```python
from build123d import *

# Parameters (mm, degrees)
F0_W     = 45.3136
F0_H     = 45.3136
F1_DEPTH = 2.3876
F2_R     = 22.6568
F2_R_2   = 19.8374
F3_DEPTH = 92.2274
F4_W     = 28.575
F4_H     = 28.575
F5_DEPTH = 4.7752
F6_R     = 21.1328
F7_DEPTH = 19.05
F8_R     = 5.08


with BuildPart() as f1:
    # F0 (on Top) → F1 (new body, symmetric)
    with BuildSketch(Plane.XY):
        Rectangle(F0_W, F0_H)
    extrude(amount=F1_DEPTH, both=True)

    # F2 (on face) → F3 (join)
    with BuildSketch(Plane.XY.offset(2.3876)):
        Circle(F2_R)
        Circle(F2_R_2, mode=Mode.SUBTRACT)
    extrude(amount=F3_DEPTH)

    # F4 (on face) → F5 (cut, through all)
    with BuildSketch(Plane(origin=(0, 0, -2.3876), x_dir=(1, 0, 0), z_dir=(0, 0, -1))):
        Rectangle(F4_W, F4_H)
    extrude(amount=-F5_DEPTH, mode=Mode.SUBTRACT)

    # F6 (on face) → F7 (cut)
    with BuildSketch(Plane.XY.offset(94.615)):
        Circle(F6_R)
    extrude(amount=-F7_DEPTH, mode=Mode.SUBTRACT)

    # F8
    f8_edges = [f1.edges().sort_by_distance(p)[0] for p in [
        (-22.6568, -22.6568, 0),
        (-22.6568, 22.6568, 0),
        (22.6568, -22.6568, 0),
        (22.6568, 22.6568, 0),
    ]]
    fillet(f8_edges, radius=F8_R)


solid = f1.part
```
Check sheet for the modelled part. Datum: model origin and axes. Units: mm. A direction names the side the tool comes from. Round coordinates to 2 decimals unless told otherwise and drop trailing zeros. Write each loop counter-clockwise with the first axis right and the second up, starting at its lowest first coordinate (ties: lowest second). Pieces come first, ordered by that corner, then holes. Notation, with made-up numbers: (28, 79.25) -> (36, 79.25) arc R22 cw to (36, 116.25) -> close; hole circle Ø5 at (75.5, 58.5). An arc over 180 degrees is marked (long way). One line per question, with ' | ' between items. Start each with the question number.
1. Sectioned sample at D-D, the plane x = 16.5. Record the cut outline in (y, z) (3 decimals), then the cut area to 3 significant figures.
2. Sectioned sample at A-A, the plane y = -12. Record the cut outline in (x, z) (1 decimal), then the cut area to 3 significant figures.
3. Release check for a two-part mould opening along X. For faces 1 (the face through (0, -22.657, 0)), 2 (the face through (-21.21, -21.13, 0.03)), 3 (the face through (-17.98, -13.786, 47.856)), 4 (the face through (14.288, 0, 0)) record: +X half, -X half, draft (parallel to the pull), parting line (faces both ways), or undercut.
4. Sectioned sample at C-C, the plane z = 40. Record the cut outline in (x, y), then the cut area to 3 significant figures.
5. Scan lines: line 1 along Y through (x, z) = (0, 38); line 2 along Y through (x, z) = (0, 82.75); line 3 along Z through (x, y) = (-18.5, -10) (3 decimals). Record each from-to range of solid material in increasing order. Write a range as from..to.
6. Set-up check for faces 5 (the face through (17, 17, 2.388)), 6 (the face through (12, -16, 75.565)), 7 (the face through (-21.13, 21.21, -0.03)), 8 (the face through (-17, -18, 2.388)): record each of +Z, -Z, +X, -X, +Y, -Y from which the full face is reachable in a straight line by a thin tool's end or side.
7. Depth check by flat-ended pin: pin 1 (1.7 mm diameter, centred on x = -17, y = 4, fed in from +Z); pin 2 (6 mm diameter, centred on x = -12.5, z = 34.5, fed in from +Y); pin 3 (10 mm diameter, centred on x = 6, z = 19.5, fed in from -Y). Enter the tip coordinate at first touch or a pass-through.
8. Sectioned sample at B-B, the plane x = 8. Record the cut outline in (y, z) (1 decimal).
Taken from the geometry:
1) outline: (-22.657, -2.388) -> (22.657, -2.388) -> (22.657, 2.388) -> (15.527, 2.388) -> (15.527, 94.615) -> (13.204, 94.615) -> (13.204, 75.565) -> (11.012, 75.565) -> (11.012, 2.388) -> (-11.012, 2.388) -> (-11.012, 75.565) -> (-13.204, 75.565) -> (-13.204, 94.615) -> (-15.527, 94.615) -> (-15.527, 2.388) -> (-22.657, 2.388) -> close | area: 966 mm^2
2) outline: (-22.7, -2.4) -> (-14.3, -2.4) -> (-14.3, 2.4) -> (-15.8, 2.4) -> (-15.8, 75.6) -> (-17.4, 75.6) -> (-17.4, 94.6) -> (-19.2, 94.6) -> (-19.2, 2.4) -> (-22.7, 2.4) -> close; (14.3, -2.4) -> (22.7, -2.4) -> (22.7, 2.4) -> (19.2, 2.4) -> (19.2, 94.6) -> (17.4, 94.6) -> (17.4, 75.6) -> (15.8, 75.6) -> (15.8, 2.4) -> (14.3, 2.4) -> close | area: 650 mm^2
3) face 1: draft | face 2: -X half | face 3: parting line | face 4: undercut
4) outline: circle Ø45.31 at (0, 0); hole circle Ø39.67 at (0, 0) | area: 376 mm^2
5) line 1: y = -22.66..-19.84, 19.84..22.66 | line 2: y = -22.66..-21.13, 21.13..22.66 | line 3: z = -2.388..75.565
6) face 5: +Z, +X, +Y | face 6: +Z | face 7: +Z, -Z, -X, +Y | face 8: +Z, -X, -Y
7) pin 1: stops at z = 2.39 | pin 2: stops at y = 20.57 | pin 3: stops at y = -22.63
8) outline: (-22.7, -2.4) -> (-14.3, -2.4) -> (-14.3, 2.4) -> (-18.2, 2.4) -> (-18.2, 75.6) -> (-19.6, 75.6) -> (-19.6, 94.6) -> (-21.2, 94.6) -> (-21.2, 2.4) -> (-22.7, 2.4) -> close; (14.3, -2.4) -> (22.7, -2.4) -> (22.7, 2.4) -> (21.2, 2.4) -> (21.2, 94.6) -> (19.6, 94.6) -> (19.6, 75.6) -> (18.2, 75.6) -> (18.2, 2.4) -> (14.3, 2.4) -> close
